Input: part model. Units: mm. Frame: model coordinates. A direction names the side the tool comes from. Round coordinates to 2 decimals unless told otherwise and drop trailing zeros. Order: outer loops, then holes, each group sorted by start corner. A loop starts at its lowest first (then second) coordinate and runs counter-clockwise, first axis right, second up. Notation, with made-up numbers: (-37, 59.5) - (13, 59.5) arc R24 cw to (13, 91.5) - close; hole circle Ø1 at (34.5, 13.25). An arc over 180 degrees is marked (long way). One line per item, written item: value. Start each with the question number.
Autodesk Inventor part; units mm, degrees
ref_plane "YZ Plane" through (0, 0, 0) normal (1, 0, 0) x (0, 1, 0)
ref_plane "XZ Plane" through (0, 0, 0) normal (0, 1, 0) x (-1, 0, 0)
ref_plane "XY Plane" through (0, 0, 0) normal (0, 0, 1) x (1, 0, 0)
sketch "Skizze1" plane through (0, 0, 0) normal (0, 0, 1) x (1, 0, 0)
  line L0 (0, 0) -> (41, 0)
  line L1 (41, 0) -> (41, 75)
  line L2 (41, 75) -> (0, 75)
  line L3 (0, 75) -> (0, 0)
  line L4 (5, 75) -> (10, 75)
  line L5 (10, 75) -> (10, 70)
  line L6 (10, 70) -> (5, 70)
  line L7 (5, 70) -> (5, 75)
  line L8 (18, 75) -> (23, 75)
  line L9 (23, 75) -> (23, 70)
  line L10 (23, 70) -> (18, 70)
  line L11 (18, 70) -> (18, 75)
  line L12 (31, 75) -> (36, 75)
  line L13 (36, 75) -> (36, 70)
  line L14 (36, 70) -> (31, 70)
  line L15 (31, 70) -> (31, 75)
  line L16 (0, 65) -> (10, 65)
  line L17 (10, 65) -> (10, 32)
  line L18 (10, 32) -> (0, 32)
  line L19 (0, 32) -> (0, 65)
  line L20 (41, 65) -> (33.5, 65)
  line L21 (33.5, 65) -> (33.5, 27)
  line L22 (33.5, 27) -> (41, 27)
  line L23 (41, 27) -> (41, 65)
  line L24 (41, 20.6907) -> (0, 25)
  point P0 (0, 32)
  dimension "d0" = 150
  dimension "d1" = 41
  dimension "d2" = 5
  dimension "d3" = 5
  dimension "d4" = 5
  dimension "d5" = 18
  dimension "d6" = 31
  dimension "d7" = 64
  dimension "d8" = 54
  dimension "d9" = 130
  dimension "d10" = 130
  dimension "d11" = 7.5
  dimension "d12" = 10
  dimension "d13" = 96
  dimension "d14" = 50
revolve "Umdrehung1" add sketch "Skizze1" angle 360 about axis through (0, 0, 0) along (1, 0, 0) contours L3 L18 L17 L16 L2 L7 L6 L5 L11 L10 L9 L15 L14 L13 L1 L20 L21 L22 L24
chamfer "Fase1" distance 3 angle 45 4 edges at (33.5, -65, 0) (33.5, -27, 0) (10, -32, 0) (10, -65, 0)
chamfer "Fase2" distance 2 angle 45 2 edges at (41, -75, 0) (0, -75, 0)
equation "\"d10\" = d9"
properties part number "Kolben" material "Stahl AISI 4130"
1. Pull-direction query (X, two-part tool) for faces 1 (the face through (41, -49, -43)), 2 (the face through (36, 50, -50)), 3 (the face through (3.55, 62, 19.52)); classes: released by +X, released by -X, zero draft, split by the parting line, or undercut.
2. Set-up query: faces 4 (the face through (3.45, -6.94, 31.24)), 5 (the face through (38.78, -5.85, -26.36)), 6 (the face through (33.465, -55.55, 42.594)). Return all of +Z, -Z, +X, -X, +Y, -Y with unobstructed straight access to the full face (end or side cutting, diameter ignored); none if empty.
3. Line query: line 1 (Z direction, x = 37.4, y = 0); line 2 (Z direction, x = 38.45, y = 0); line 3 (X direction, y = 49, z = 56). Output: solid intervals per line, ascending. Write a range as from..to.
4. Pin query (flat end, axial travel): pin 1 (4 mm diameter, centred on x = 13.5, z = 55.5, fed in from -Y); pin 2 (4 mm diameter, centred on x = 27.5, y = 20.5, fed in from +Z); pin 3 (12 mm diameter, centred on y = 56, z = 25.5, fed in from +X); pin 4 (1 mm diameter, centred on y = -38, z = 29.5, fed in from -X). Return the tip coordinate at first contact, or that it passes through.
5. Section A-A (x = 29). Return the cut outline in (y, z), then the cut area to 3 significant figures.
Solved:
1. face 1: released by +X
1. face 2: undercut
1. face 3: zero draft
2. face 4: -X
2. face 5: +X
2. face 6: none
3. line 1: z = -75..-65, -27..-21.07, 21.07..27, 65..75
3. line 2: z = -75..-65, -27..-20.96, 20.96..27, 65..75
3. line 3: x = 1.41..5, 10..18, 23..31, 36..39.59
4. pin 1: stops at y = -52.56
4. pin 2: stops at z = 72.68
4. pin 3: stops at x = 41
4. pin 4: stops at x = 10
5. outline: circle Ø150 at (0, 0); hole circle Ø43.9 at (0, 0)
5. area: 16,200 mm²
